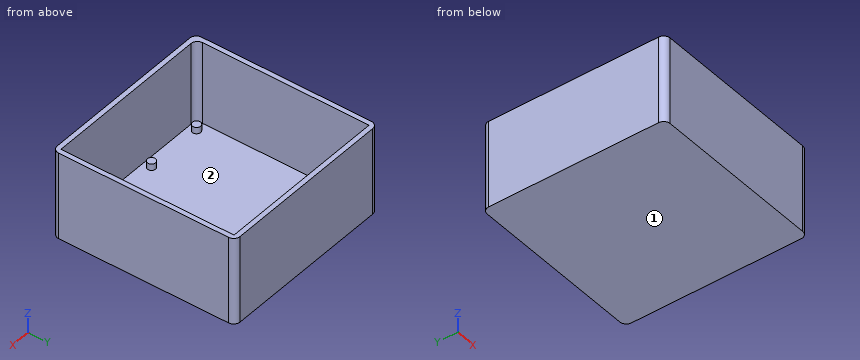
from build123d import *

# Parameters (mm, degrees)
F0_W     = 53.34
F0_H     = 53.34
F1_DEPTH = 25.4
F2_T     = 1.5
F3_R     = 1.27
F3_R_2   = 1.143
F4_DEPTH = 2
F5_R     = 2


# Not quite as in the source:
# - two fillets or chamfers of one size are made in one step


with BuildPart() as f1:
    # F0 (on Top) → F1 (new body)
    with BuildSketch(Plane.XY):
        Rectangle(F0_W, F0_H)
    extrude(amount=F1_DEPTH)

    # F2
    f2_openings = [f1.faces().sort_by_distance(p)[0] for p in [
        (0, 0, 25.4),
    ]]
    offset(amount=F2_T, openings=f2_openings, kind=Kind.INTERSECTION)

    # F3 (on face) → F4 (join)
    with BuildSketch(Plane.XY):
        with Locations((-23.63, -24.13)):
            Circle(F3_R)
        with Locations((-5.85, -24.13)):
            Circle(F3_R)
        with Locations((-24.253, 21.59)):
            Circle(F3_R_2)
        with Locations((-5.203, 21.59)):
            Circle(F3_R_2)
    extrude(amount=F4_DEPTH)

    # F5
    f5_edges = [f1.edges().sort_by_distance(p)[0] for p in [
        (-26.67, -26.67, 12.7),
        (28.17, -28.17, 11.95),
        (-28.17, -28.17, 11.95),
        (28.17, 28.17, 11.95),
        (-28.17, 28.17, 11.95),
    ]]
    fillet(f5_edges, radius=F5_R)


solid = f1.part
Work out the finished part from the listing and answer in its coordinate system (mm). Face numbers are marked on the shaded views. A direction names the side the tool comes from. Coordinates: 2 decimals unless noted, no trailing zeros. Write each loop counter-clockwise with the first axis right and the second up, starting at its lowest first coordinate (ties: lowest second). Pieces come first, ordered by that corner, then holes. Notation, with made-up numbers: M -17.5,80.25 L 25.5,80.25 A16 ccw 25.5,94.25 Z; hole C 39.25,-6.75 d9. An arc over 180 degrees is marked long. Use one line per item in the form item = value. Start each with the question number.
1. Straight lines are drawn through the part: probe 1 along X at (y, z) = (-24, 15); probe 2 along Z at (x, y) = (-17, 11). For each, find the intervals that lie inside material, in ascending order. Write a range as from..to.
2. The part is cut by section C-C (y = 21.59). Give the vertices of the cut face in (x, z).
3. The part is cut by section A-A (z = 0.75). Give the vertices of the cut face in (x, y).
4. The part is cut by section D-D (x = 2). Give the vertices of the cut face in (y, z).
5. Each of these flat-tipped pins is pushed along its axis until it touches: P1, Ø2, axis at x = -24, y = -24, coming from the +Z side; P2, Ø8, axis at x = 16.5, y = -18.5, coming from the +Z side. Where does it stop, or does it pass through?
6. The part is cut by section B-B (z = 9.25). Give the vertices of the cut face in (x, y), plus the area to 3 significant figures.
7. A tool of negligible diameter and unlimited length cuts with its end or side. For the marked faces 1 and 2, from which of +Z, -Z, +X, -X, +Y, -Y can it reach the whole face along a straight path? Write none if from no direction.
Evaluation:
q1.probe_1 = -28.17..-26.67, 26.67..28.17
q1.probe_2 = -1.5..0
q2.outline = M -28.17,-1.5 L 28.17,-1.5 L 28.17,25.4 L 26.67,25.4 L 26.67,0 L -4.06,0 L -4.06,2 L -6.35,2 L -6.35,0 L -23.11,0 L -23.11,2 L -25.4,2 L -25.4,0 L -26.67,0 L -26.67,25.4 L -28.17,25.4 Z
q3.outline = M -28.17,-26.17 A2 ccw -26.17,-28.17 L 26.17,-28.17 A2 ccw 28.17,-26.17 L 28.17,26.17 A2 ccw 26.17,28.17 L -26.17,28.17 A2 ccw -28.17,26.17 Z; C -24.25,21.59 d2.29; C -23.63,-24.13 d2.54; C -5.85,-24.13 d2.54; C -5.2,21.59 d2.29; hole M -26.67,-24.67 A2 ccw -24.67,-26.67 L 26.67,-26.67 L 26.67,26.67 L -26.67,26.67 Z
q4.outline = M -28.17,-1.5 L 28.17,-1.5 L 28.17,25.4 L 26.67,25.4 L 26.67,0 L -26.67,0 L -26.67,25.4 L -28.17,25.4 Z
q5.P1 = 2
q5.P2 = 0
q6.outline = M -28.17,-26.17 A2 ccw -26.17,-28.17 L 26.17,-28.17 A2 ccw 28.17,-26.17 L 28.17,26.17 A2 ccw 26.17,28.17 L -26.17,28.17 A2 ccw -28.17,26.17 Z; hole M -26.67,-24.67 A2 ccw -24.67,-26.67 L 26.67,-26.67 L 26.67,26.67 L -26.67,26.67 Z
q6.area = 326 mm^2
q7.face_1 = -Z, +X, -X, +Y, -Y
q7.face_2 = +Z
